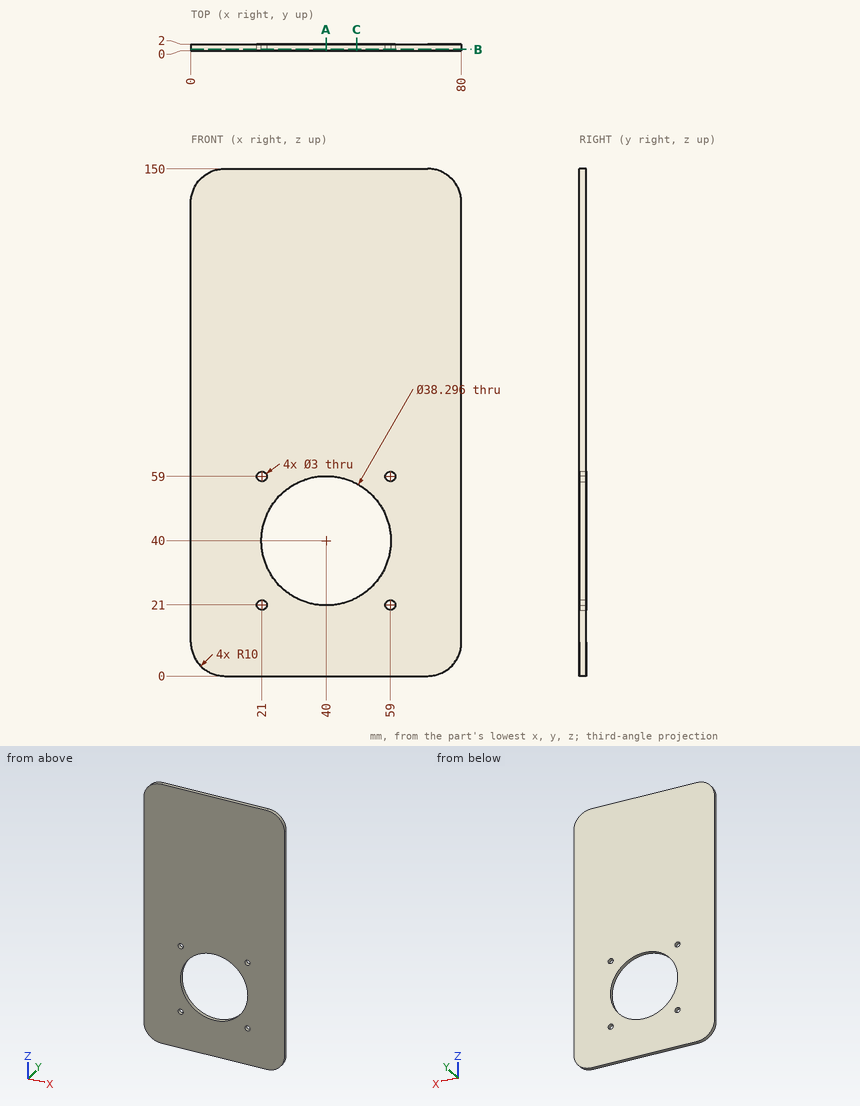
Design review of the part shown in the three views and the two pictorial views. Dimensions are in mm from the part's minimum x, y and z. Give positions to 0.01 mm unless a question says otherwise; leave off trailing zeros. Loops run counter-clockwise (first coordinate to the right, second up) from the corner with the lowest first, then second, coordinate; pieces in that order, holes last. Notation, with made-up numbers: M 42,-34.75 L 65,-34.75 A16 ccw 65,-7.75 Z; hole C 24,59.5 d10. An arc over 180 degrees is marked long. Answer as a JSON object with one key per item and string values.
Item 1: We need section A-A (x = 40). State the section outline as (y, z) points.
Output values:
{"outline": "M 0,0 L 2,0 L 2,20.85 L 0,20.85 Z; M 0,59.15 L 2,59.15 L 2,150 L 0,150 Z"}
Item 2: Wall thickness on line 1 along Z through (x, y) = (20.5, 0.65); line 2 along Z through (x, y) = (41, 1.65); line 3 along X through (y, z) = (0.95, 40): over which ranges is each line inside the solid? List them lowest first.
Output values:
{"line 1": "z = 0 to 19.59, 22.41 to 57.59, 60.41 to 150", "line 2": "z = 0 to 20.88, 59.12 to 150", "line 3": "x = 0 to 20.85, 59.15 to 80"}
Item 3: We need section B-B (y = 0.4). State the section outline as (x, z) points, and give its area (3 significant figures).
Output values:
{"outline": "M 0,10 A10 ccw 10,0 L 70,0 A10 ccw 80,10 L 80,140 A10 ccw 70,150 L 10,150 A10 ccw 0,140 Z; hole C 21,21 d3; hole C 21,59 d3; hole C 40,40 d38.3; hole C 59,21 d3; hole C 59,59 d3", "area": "10,700 mm2"}
Item 4: We need section C-C (x = 49). State the section outline as (y, z) points.
Output values:
{"outline": "M 0,0 L 2,0 L 2,23.1 L 0,23.1 Z; M 0,56.9 L 2,56.9 L 2,150 L 0,150 Z"}
Item 5: For P1, Ø2.5, axis at x = 21, z = 21, coming from the -Y side, flat-tipped, find the tip position at first contact; note if it passes through.
Output values:
{"P1": "passes through"}
